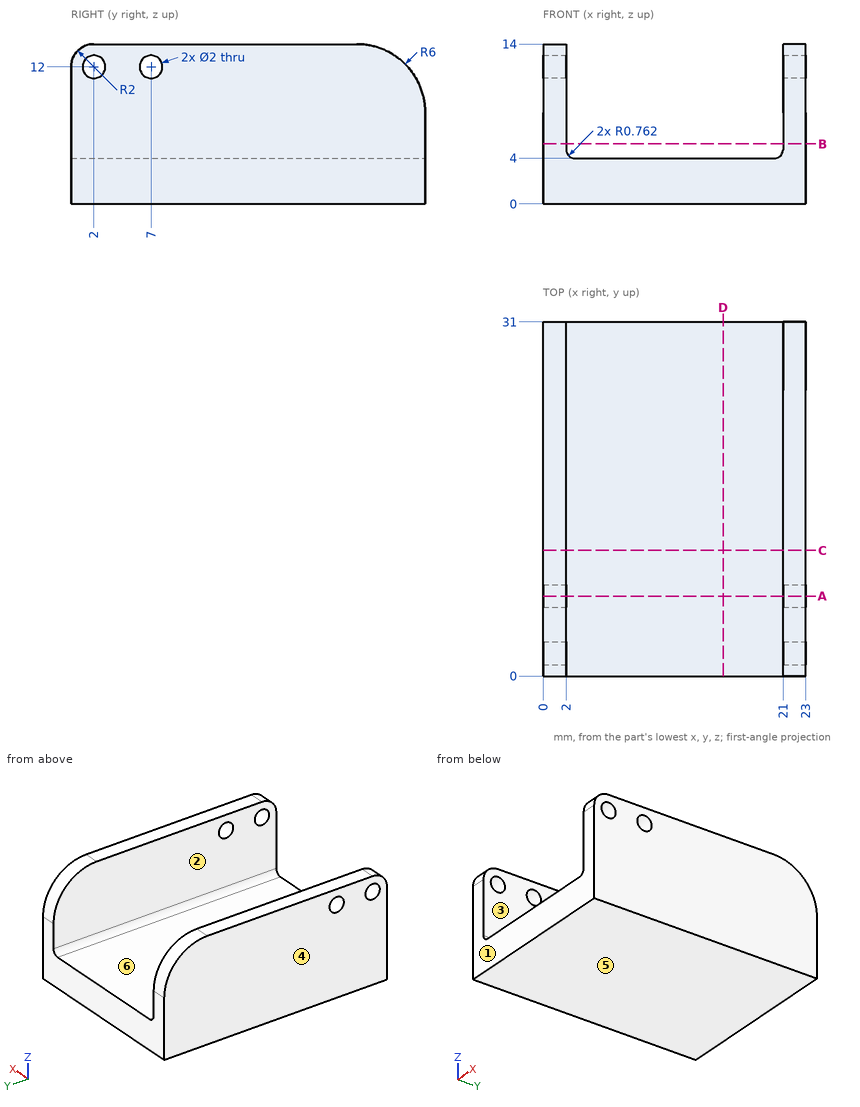
Job drawing, mm, ordinate dimensions from the low corner. One solid piece. A direction names the side the tool comes from. Round coordinates to 2 decimals unless told otherwise and drop trailing zeros. Loops run counter-clockwise (first coordinate to the right, second up) from the corner with the lowest first, then second, coordinate; pieces in that order, holes last.
(1) Drop a flat-ended pin along its axis: pin 1 (1 mm diameter, centred on x = 15.5, y = 27.5, fed in from +Z). Give the stop position or say it passes through.
(2) Two-plate mould, pull along X, no slides. Class the marked faces 1, 2, 3 and 4: +X half, -X half, draft (parallel to the pull), parting line (faces both ways), or undercut.
(3) Cut at D-D (x = 15.75). Give the cut face in (y, z).
(4) Cut at C-C (y = 11). Give the cut face in (x, z).
(5) Which spindle directions (+Z, -Z, +X, -X, +Y, -Y) get a long thin tool onto all of the face, cutting with end or side? Do the marked faces 5 and 6. Say none if no direction does.
(6) Wall check: line 1 along X through (y, z) = (26, 6.25); line 2 along Y through (x, z) = (0.5, 12); line 3 along Z through (x, y) = (4.5, 28). Give the ranges that are in metal, low to high.
(7) Cut at A-A (y = 7). Give the cut face in (x, z), plus the area to 3 significant figures.
(8) Cut at B-B (z = 5.25). Give the cut face in (x, y).
Findings below:
1. pin 1: stops at z = 4
2. face 1: draft
2. face 2: undercut
2. face 3: undercut
2. face 4: -X half
3. outline: (0, 0) - (31, 0) - (31, 4) - (0, 4) - close
4. outline: (0, 0) - (23, 0) - (23, 14) - (21, 14) - (21, 4.76) arc R0.76 cw to (20.24, 4) - (2.76, 4) arc R0.76 cw to (2, 4.76) - (2, 14) - (0, 14) - close
5. face 5: -Z, +X, -X, +Y, -Y
5. face 6: +Z, +Y, -Y
6. line 1: x = 0 to 2, 21 to 23
6. line 2: y = 0 to 1, 3 to 6, 8 to 29.47
6. line 3: z = 0 to 4
7. outline: (0, 0) - (23, 0) - (23, 11) - (21, 11) - (21, 4.76) arc R0.76 cw to (20.24, 4) - (2.76, 4) arc R0.76 cw to (2, 4.76) - (2, 11) - (0, 11) - close; (0, 13) - (2, 13) - (2, 14) - (0, 14) - close; (21, 13) - (23, 13) - (23, 14) - (21, 14) - close
7. area: 124 mm2
8. outline: (0, 0) - (2, 0) - (2, 31) - (0, 31) - close; (21, 0) - (23, 0) - (23, 31) - (21, 31) - close
